Input: part model. Units: mm. Frame: model coordinates. Coordinates: 2 decimals unless noted, no trailing zeros. Order: outer loops, then holes, each group sorted by start corner. A loop starts at its lowest first (then second) coordinate and runs counter-clockwise, first axis right, second up. Notation, with made-up numbers: (35, 87) - (71, 87) arc R15 cw to (71, 93) - close; hole circle Ø1 at (-12, 69). An arc over 180 degrees is marked (long way). Use a Markdown table: item, result. Add a question column.
from build123d import *

# Parameters (mm, degrees)
CROQUIS1_W              = 250
CROQUIS1_H              = 280
CROQUIS1_R              = 44.5
CROQUIS1_W_2            = 96.425
CROQUIS1_H_2            = 216.5
CROQUIS1_H_3            = 110.55
SALIENTE_EXTRUIR1_DEPTH = 12.7
CROQUIS2_W              = 37.2
CROQUIS2_H              = 12.7
CROQUIS2_W_2            = 74.4
CORTAR_EXTRUIR1_DEPTH   = 13.7


with BuildPart() as part:
    # Croquis1 → Saliente-Extruir1 (new body)
    with BuildSketch(Plane.XY):
        Rectangle(CROQUIS1_W, CROQUIS1_H)
        with Locations((62.5, 64.8)):
            Circle(CROQUIS1_R, mode=Mode.SUBTRACT)
        with Locations((-57.7375, 0)):
            Rectangle(CROQUIS1_W_2, CROQUIS1_H_2, mode=Mode.SUBTRACT)
        with Locations((57.7375, -52.975)):
            Rectangle(CROQUIS1_W_2, CROQUIS1_H_3, mode=Mode.SUBTRACT)
    extrude(amount=SALIENTE_EXTRUIR1_DEPTH)

    # Croquis2 → Cortar-Extruir1 (cut, through all)
    with BuildSketch(Plane.XY.offset(12.7)):
        with Locations((-106.4, 133.65)):
            Rectangle(CROQUIS2_W, CROQUIS2_H)
        with Locations((0, 133.65)):
            Rectangle(CROQUIS2_W_2, CROQUIS2_H)
        with Locations((106.4, 133.65)):
            Rectangle(CROQUIS2_W, CROQUIS2_H)
        with BuildLine():
            Line((-117.475, 120.95), (-113.475, 120.95))
            ThreePointArc((-113.475, 120.95), (-110.275, 117.75), (-113.475, 114.55))
            Line((-113.475, 114.55), (-117.475, 114.55))
            ThreePointArc((-117.475, 114.55), (-120.675, 117.75), (-117.475, 120.95))
        make_face()
        with BuildLine():
            Line((-2, 120.95), (2, 120.95))
            ThreePointArc((2, 120.95), (5.2, 117.75), (2, 114.55))
            Line((2, 114.55), (-2, 114.55))
            ThreePointArc((-2, 114.55), (-5.2, 117.75), (-2, 120.95))
        make_face()
        with BuildLine():
            Line((113.475, 120.95), (117.475, 120.95))
            ThreePointArc((117.475, 120.95), (120.675, 117.75), (117.475, 114.55))
            Line((117.475, 114.55), (113.475, 114.55))
            ThreePointArc((113.475, 114.55), (110.275, 117.75), (113.475, 120.95))
        make_face()
    cortar_extruir1 = extrude(amount=-CORTAR_EXTRUIR1_DEPTH, mode=Mode.SUBTRACT)

    # Simetría1: Cortar-Extruir1 across plane
    add(cortar_extruir1.mirror(Plane.ZX), mode=Mode.SUBTRACT)


solid = part.part
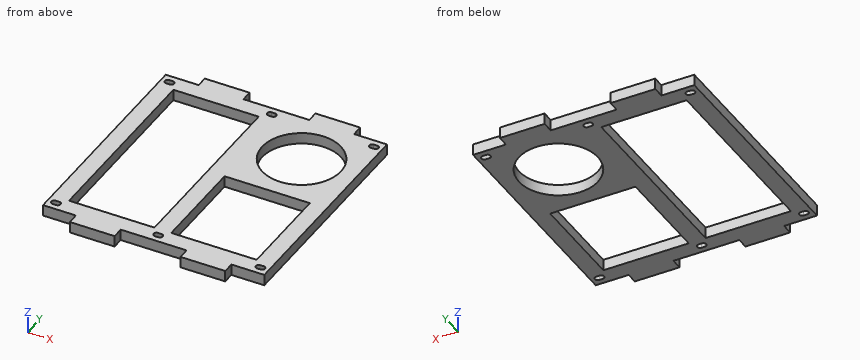
1) Cut plane B-B (x = 62.5). Return the cut outline in (y, z), and give its area (3 significant figures).
2) Contact query for flat-ended pins moving along their axis: P1, Ø3, axis at x = 115.5, z = 4, coming from the +Y side; P2, Ø1.2, axis at x = 1, z = 3, coming from the -Y side; P3, Ø12, axis at x = 49, y = 96, coming from the -Z side. Output: stop coordinate, or through.
3) Material intervals for L1, parallel to X at y = -75.5, z = 4 (3 decimals); L2, parallel to Y at x = -114.5, z = 4.5; L3, parallel to Y at x = 62.5, z = 6, sorted ascending.
4) Cut plane C-C (y = -117.75). Return the cut outline in (x, z) (3 decimals).
5) Cut plane A-A (y = -69.5). Return the cut outline in (x, z) (3 decimals).
6) Cut plane D-D (x = -83.5). Return the cut outline in (y, z).
Computed:
| question | item | result |
|---|---|---|
| 1 | outline | (-140, 0) - (-108.25, 0) - (-108.25, 12.7) - (-140, 12.7) - close; (2.3, 0) - (20.3, 0) - (20.3, 12.7) - (2.3, 12.7) - close; (109.3, 0) - (140, 0) - (140, 12.7) - (109.3, 12.7) - close |
| 1 | area | 1,020 mm2 |
| 2 | P1 | stops at y = 127.3 |
| 2 | P2 | stops at y = -127.3 |
| 2 | P3 | passes through |
| 3 | L1 | x = -125 to -105.95, -9.525 to 9.525, 105.95 to 125 |
| 3 | L2 | y = -127.3 to -120.95, -114.55 to 114.55, 120.95 to 127.3 |
| 3 | L3 | y = -140 to -108.25, 2.3 to 20.3, 109.3 to 140 |
| 4 | outline | (-125, 0) - (-120.675, 0) - (-120.675, 12.7) - (-125, 12.7) - close; (-110.275, 0) - (-5.2, 0) - (-5.2, 12.7) - (-110.275, 12.7) - close; (5.2, 0) - (110.275, 0) - (110.275, 12.7) - (5.2, 12.7) - close; (120.675, 0) - (125, 0) - (125, 12.7) - (120.675, 12.7) - close |
| 5 | outline | (-125, 0) - (-105.95, 0) - (-105.95, 12.7) - (-125, 12.7) - close; (-9.525, 0) - (9.525, 0) - (9.525, 12.7) - (-9.525, 12.7) - close; (105.95, 0) - (125, 0) - (125, 12.7) - (105.95, 12.7) - close |
| 6 | outline | (-140, 0) - (-108.25, 0) - (-108.25, 12.7) - (-140, 12.7) - close; (108.25, 0) - (140, 0) - (140, 12.7) - (108.25, 12.7) - close |
